Here's the drawing with two shaded views (mm, measured from the low corner). I have some questions. A direction names the side the tool comes from. Give positions to 0.01 mm unless a question says otherwise; leave off trailing zeros. Write each loop counter-clockwise with the first axis right and the second up, starting at its lowest first coordinate (ties: lowest second). Pieces come first, ordered by that corner, then holes.
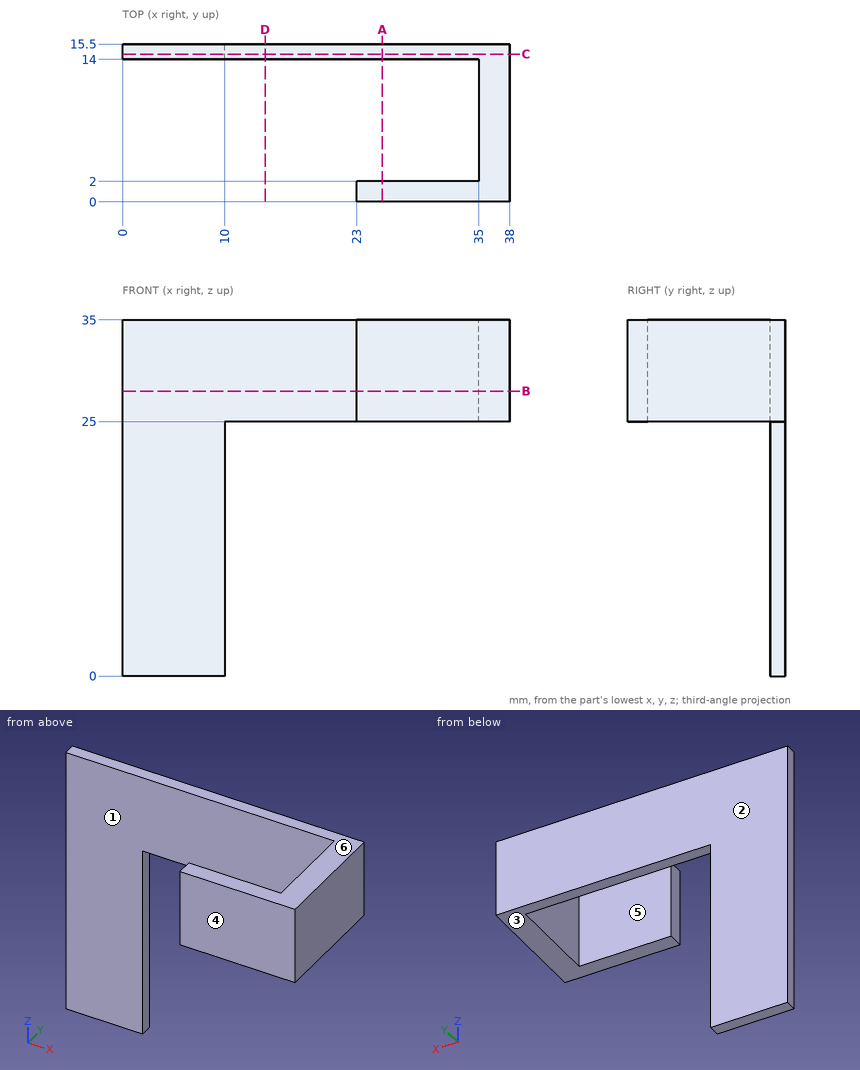
1) For the marked faces 1, 2 and 3, which set-ups out of +Z, -Z, +X, -X, +Y, -Y let a thin tool reach every point of the face, with its end or its side?
Values follow:
face 1: +Z, -Z, -X
face 2: +Z, -Z, +X, -X, +Y
face 3: -Z, +X, +Y, -Y
2) Suppose I cut it at A-A on x = 25.5. Write out the boundary of the cut face in (y, z), plus the area to 3 significant figures.
Values follow:
outline: (0, 25) - (2, 25) - (2, 35) - (0, 35) - close; (14, 25) - (15.5, 25) - (15.5, 35) - (14, 35) - close
area: 35.0 mm2
3) Suppose I cut it at B-B on z = 28. Write out the boundary of the cut face in (x, y), plus the area to 3 significant figures.
Values follow:
outline: (0, 14) - (35, 14) - (35, 2) - (23, 2) - (23, 0) - (38, 0) - (38, 15.5) - (0, 15.5) - close
area: 123 mm2
4) If we mould it in two halves opening along Y, with no side actions, what happens to the marked faces 4, 5 and 6? For each: +Y half, -Y half, draft (parallel to the pull), parting line (faces both ways), or undercut.
Values follow:
face 4: -Y half
face 5: undercut
face 6: draft
5) Suppose I cut it at C-C on y = 14.5. Write out the boundary of the cut face in (x, z), plus the area to 3 significant figures.
Values follow:
outline: (0, 0) - (10, 0) - (10, 25) - (38, 25) - (38, 35) - (0, 35) - close
area: 630 mm2
6) Suppose I cut it at D-D on x = 14. Write out the boundary of the cut face in (y, z), plus the area to 3 significant figures.
Values follow:
outline: (14, 25) - (15.5, 25) - (15.5, 35) - (14, 35) - close
area: 15.0 mm2
7) For pin 1 Ø3 at (y, z) = (10, 29) entering from -X; pin 2 Ø5 at (y, z) = (3.5, 29) entering from -X; pin 3 Ø1.6 at (y, z) = (14.5, 9) entering from +X, each with a flat end and sliding along its axis, tell me the tip position at first contact or that it passes through.
Values follow:
pin 1: stops at x = 35
pin 2: stops at x = 23
pin 3: stops at x = 10
8) Please list where these lines run through material, in increasing order: L1, parallel to Z at x = 36, y = 11.5; L2, parallel to Y at x = 31.5, z = 33; L3, parallel to X at y = 13, z = 32.5.
Values follow:
L1: z = 25 to 35
L2: y = 0 to 2, 14 to 15.5
L3: x = 35 to 38
